Source: CAD feature listing. Evaluate the final solid. Frame: model axes, mm. A direction names the side the tool comes from. Coordinates: 2 decimals unless noted, no trailing zeros. Loops run counter-clockwise (first coordinate to the right, second up) from the corner with the lowest first, then second, coordinate; pieces in that order, holes last. Notation, with made-up numbers: (53.25, -39) - (96.25, -39) arc R27 cw to (96.25, -11) - close; hole circle Ø1 at (-2.5, 72). An arc over 180 degrees is marked (long way). Write item = value, one per line. Start each with the question number.
Autodesk Inventor part; units mm, degrees
ref_plane "YZ Plane" through (0, 0, 0) normal (1, 0, 0) x (0, 1, 0)
ref_plane "XZ Plane" through (0, 0, 0) normal (0, 1, 0) x (-1, 0, 0)
ref_plane "XY Plane" through (0, 0, 0) normal (0, 0, 1) x (1, 0, 0)
sketch "Sketch1" plane through (0, 0, 0) normal (0, 1, 0) x (-1, 0, 0)
  line L0 (0, 0) -> (70, 0)
  line L1 (70, 0) -> (70, -110)
  line L2 (70, -110) -> (0, -110)
  line L3 (0, -110) -> (0, 0)
  line L4 (2.5, -2.49) -> (67.5, -2.49)
  line L5 (67.5, -2.49) -> (67.5, -107.49)
  line L6 (67.5, -107.49) -> (2.5, -107.49)
  line L7 (2.5, -107.49) -> (2.5, -2.49)
  line L8 (67.5, -54.99) -> (2.5, -54.99) construction
  line L9 (67.5, -54.99) -> (63.6, -54.99) construction
  line L10 (63.6, -54.99) -> (63.6, -71.2) construction
  line L11 (63.6, -71.2) -> (67.5, -71.2) construction
  line L12 (67.5, -71.2) -> (67.5, -54.99) construction
  line L13 (63.6, -68.2) -> (63.6, -74.2) construction
  line L14 (62.35, -68.2) -> (62.35, -74.2)
  line L15 (64.85, -74.2) -> (64.85, -68.2)
  arc A0 (64.85, -68.2) -> (62.35, -68.2) centre (63.6, -68.2) ccw
  arc A1 (62.35, -74.2) -> (64.85, -74.2) centre (63.6, -74.2) ccw
  line L16 (63.6, -71.2) -> (63.6, -87.6) construction
  line L17 (2.5, -87.6) -> (6.05, -87.6) construction
  line L18 (6.05, -84.6) -> (6.05, -90.6) construction
  line L19 (4.8, -84.6) -> (4.8, -90.6)
  line L20 (7.3, -90.6) -> (7.3, -84.6)
  arc A2 (7.3, -84.6) -> (4.8, -84.6) centre (6.05, -84.6) ccw
  arc A3 (4.8, -90.6) -> (7.3, -90.6) centre (6.05, -90.6) ccw
  line L21 (67.5, -2.49) -> (63.6, -2.49) construction
  line L22 (63.6, -2.49) -> (63.6, -18.7) construction
  line L23 (63.6, -18.7) -> (67.5, -18.7) construction
  line L24 (67.5, -18.7) -> (67.5, -2.49) construction
  line L25 (63.6, -18.7) -> (63.6, -35.1) construction
  line L26 (2.5, -35.1) -> (6.05, -35.1) construction
  line L27 (63.6, -15.7) -> (63.6, -21.7) construction
  line L28 (62.35, -15.7) -> (62.35, -21.7)
  line L29 (64.85, -21.7) -> (64.85, -15.7)
  arc A4 (64.85, -15.7) -> (62.35, -15.7) centre (63.6, -15.7) ccw
  arc A5 (62.35, -21.7) -> (64.85, -21.7) centre (63.6, -21.7) ccw
  line L30 (6.05, -32.1) -> (6.05, -38.1) construction
  line L31 (4.8, -32.1) -> (4.8, -38.1)
  line L32 (7.3, -38.1) -> (7.3, -32.1)
  arc A6 (7.3, -32.1) -> (4.8, -32.1) centre (6.05, -32.1) ccw
  arc A7 (4.8, -38.1) -> (7.3, -38.1) centre (6.05, -38.1) ccw
  point P0 (35, -55)
  dimension "d0" = 70
  dimension "d1" = 110
  dimension "d2" = 65
  dimension "d3" = 105
  dimension "d4" = 52.5
  dimension "d5" = 52.5
  dimension "d6" = 3.9
  dimension "d7" = 16.21
  dimension "d8" = 3
  dimension "d9" = 2.5
  dimension "d10" = 16.4
  dimension "d11" = 3.55
  dimension "d12" = 3
  dimension "d13" = 2.5
  dimension "d14" = 19.89
  dimension "d15" = 16.4
  dimension "d16" = 3.9
  dimension "d17" = 16.21
  dimension "d18" = 16.4
  dimension "d19" = 3.55
  dimension "d20" = 3
  dimension "d21" = 2.5
  dimension "d22" = 3
  dimension "d23" = 2.5
extrude "Extrusion1" add sketch "Sketch1" along normal blind 25 contours L0 L1 L2 L3
extrude "Extrusion2" add sketch "Sketch1" along normal blind 5 contours L4 L5 L6 L7
sketch "Sketch2" plane through (0, 0, 0) normal (0, -1, 0) x (1, 0, 0)
  line L0 (-63.6, -21.7) -> (-63.6, -15.7) construction
  line L1 (-61.6, -21.7) -> (-61.6, -15.7)
  line L2 (-65.6, -15.7) -> (-65.6, -21.7)
  arc A0 (-65.6, -21.7) -> (-61.6, -21.7) centre (-63.6, -21.7) ccw
  arc A1 (-61.6, -15.7) -> (-65.6, -15.7) centre (-63.6, -15.7) ccw
  line L3 (-6.0099, -38.1033) -> (-6.0099, -32.1033) construction
  line L4 (-4.0099, -38.1033) -> (-4.0099, -32.1033)
  line L5 (-8.0099, -32.1033) -> (-8.0099, -38.1033)
  arc A2 (-8.0099, -38.1033) -> (-4.0099, -38.1033) centre (-6.0099, -38.1033) ccw
  arc A3 (-4.0099, -32.1033) -> (-8.0099, -32.1033) centre (-6.0099, -32.1033) ccw
  line L6 (-63.6, -74.2793) -> (-63.6, -68.2793) construction
  line L7 (-61.6, -74.2793) -> (-61.6, -68.2793)
  line L8 (-65.6, -68.2793) -> (-65.6, -74.2793)
  arc A4 (-65.6, -74.2793) -> (-61.6, -74.2793) centre (-63.6, -74.2793) ccw
  arc A5 (-61.6, -68.2793) -> (-65.6, -68.2793) centre (-63.6, -68.2793) ccw
  line L9 (-6.0099, -90.6) -> (-6.0099, -84.6) construction
  line L10 (-4.8, -90.6) -> (-4.8, -84.6)
  line L11 (-4.0099, -90.6) -> (-4.0099, -84.6)
  line L12 (-8.0099, -84.6) -> (-8.0099, -90.6)
  arc A6 (-8.0099, -90.6) -> (-4.0099, -90.6) centre (-6.0099, -90.6) ccw
  arc A7 (-4.0099, -84.6) -> (-8.0099, -84.6) centre (-6.0099, -84.6) ccw
  line L13 (-6.0099, -87.6) -> (-0.0099, -87.6) construction
  point P0 (0, 0)
  point P1 (-63.6, -18.7)
  point P2 (-6.0099, -35.1033)
  point P3 (-63.6, -71.2793)
  dimension "d28" = 3
  dimension "d29" = 4
  dimension "d30" = 3
  dimension "d31" = 4
  dimension "d32" = 3
  dimension "d33" = 4
  dimension "d34" = 3
  dimension "d35" = 90
  dimension "d36" = 4
extrude "Extrusion3" cut sketch "Sketch2" against normal blind 1
sketch "Sketch3" plane through (0, 25, 0) normal (0, 1, 0) x (1, 0, 0)
  line L0 (-67.5, 2.49) -> (-67.5, 107.49)
  circle A0 centre (-67.5, 2.49) radius 2.5
  line L1 (-70, 2) -> (-70, 108)
  circle A1 centre (-67.5, 107.477) radius 2.5
  line L2 (-67.5, 107.49) -> (-2.5, 107.49)
  circle A2 centre (-2.5, 107.49) radius 2.5
  point P0 (0, 0)
  dimension "d40" = 5
extrude "Extrusion4" add sketch "Sketch3" against normal blind 24 contours A2 | A0 | A1 L2 L0 | L0 L2 A1
sketch "Sketch5" plane through (0, 0, 0) normal (0, -1, 0) x (1, 0, 0)
  arc A0 (-2.5, -104.99) -> (-5, -107.49) centre (-2.5, -107.49) ccw
  arc A1 (-65, -107.49) -> (-67.5, -104.977) centre (-67.5, -107.477) ccw
  arc A2 (-67.5, -4.99) -> (-65, -2.49) centre (-67.5, -2.49) ccw
  point P0 (0, 0)
hole "Hole1" at (-2.5, 0, -107.49) at (-67.5, 0, -107.477) at (-67.5, 0, -2.49) direction (0, 1, 0) diameter 3 depth 40 tip angle 118 counterbore diameter 3.5 counterbore depth 2
fillet "Fillet2" radius 2 4 edges at (-70, 12.5, 0) (-70, 12.5, -110) (0, 12.5, -110) (0, 12.5, 0)
sketch "Sketch6" plane through (0, 0, 0) normal (0, -1, 0) x (1, 0, 0)
  line L0 (-19.0093, -31.0437) -> (-19.0093, -43.6077) construction
  line L1 (-19.0093, -43.6077) -> (-93.3266, -43.6077) construction
  line L2 (-93.3266, -43.6077) -> (-93.3266, -31.0437) construction
  line L3 (-93.3266, -31.0437) -> (-19.0093, -31.0437) construction
  line L4 (-32.1283, -26.5619) -> (-32.1283, -53.8239) construction
  line L5 (-32.1283, -53.8239) -> (-124.1375, -53.8239) construction
  line L6 (-124.1375, -53.8239) -> (-124.1375, -26.5619) construction
  line L7 (-124.1375, -26.5619) -> (-32.1283, -26.5619) construction
  line L8 (-45.7196, -50.7865) -> (-45.7196, -85.058) construction
  line L9 (-45.7196, -85.058) -> (-48.896, -85.058) construction
  line L10 (-48.896, -85.058) -> (-48.896, -50.7865) construction
  line L11 (-48.896, -50.7865) -> (-45.7196, -50.7865) construction
  point P0 (0, 0)
properties part number "SUPERIOR MODEL2"
Item 1: Cut plane C-C (x = -51.5). Return the cut outline in (y, z), then the cut area to 3 significant figures.
Item 2: Cut plane B-B (z = -88.5). Return the cut outline in (x, y), then the cut area to 3 significant figures.
Item 3: First-contact query: pin 1 (5 mm diameter, centred on x = -19.5, y = 9, fed in from +Z); pin 2 (12 mm diameter, centred on x = -52, z = -39.5, fed in from +Y); pin 3 (1.8 mm diameter, centred on x = -3, z = -108, fed in from -Y). Flat tips, straight axial feed; report the tip coordinate or a pass-through.
Item 4: Material intervals for L1, parallel to X at y = 0.75, z = -107.49; L2, parallel to Z at x = -11, y = 18; L3, parallel to X at y = 19.5, z = -74.5, sorted ascending. Write a range as [from, to].
Item 5: Draft query along X for faces 1 (the cylindrical face through (-69.4, 12.68, -109.43)), 2 (the cylindrical face through (-0.6, 12.68, -0.57)), 3 (the flat face through (-62.35, 3, -71)). Return one class per face: released by +X, released by -X, zero draft, split by the parting line, or undercut.
Item 6: Cut plane A-A (y = 9.75). Return the cut outline in (x, z), then the cut area to 3 significant figures.
Item 7: Cut plane D-D (z = -25). Return the cut outline in (x, y).
Item 8: Reachability of faces 4 (the cylindrical face through (-6, 0.5, -82.6)), 5 (the cylindrical face through (-65.75, 15.14, -105.69)), 6 (the flat face through (-4.8, 3, -35)) from +Z, -Z, +X, -X, +Y, -Y: full face, straight path, thin tool, end or side. Return the list, or none.
Responses:
q1.outline = (0, -110) - (25, -110) - (25, -107.49) - (5, -107.49) - (5, -2.49) - (25, -2.49) - (25, 0) - (0, 0) - close
q1.area = 650 mm2
q2.outline = (-70, 0) - (-8.01, 0) - (-8.01, 1) - (-7.3, 1) - (-7.3, 5) - (-67.5, 5) - (-67.5, 25) - (-70, 25) - close; (-4.8, 1) - (-4.01, 1) - (-4.01, 0) - (0, 0) - (0, 25) - (-2.5, 25) - (-2.5, 5) - (-4.8, 5) - close
q2.area = 436 mm2
q3.pin_1 = 0
q3.pin_2 = 5
q3.pin_3 = 2
q4.L1 = [-70, -69.25], [-65.75, -4.25], [-0.75, 0]
q4.L2 = [-110, -107.49], [-2.49, 0]
q4.L3 = [-70, -67.5], [-2.5, 0]
q5.face_1 = released by -X
q5.face_2 = released by +X
q5.face_3 = undercut
q6.outline = (-70, -108) arc R2 ccw to (-68, -110) - (-2, -110) arc R2 ccw to (0, -108) - (0, -2) arc R2 ccw to (-2, 0) - (-67.28, 0) arc R2.5 ccw to (-67.72, 0) - (-68, 0) arc R2 ccw to (-70, -2) - close; hole circle Ø3 at (-67.5, -107.48); hole circle Ø3 at (-67.5, -2.49); hole (-67.5, -104.98) arc R2.5 cw to (-65, -107.49) - (-5, -107.49) arc R2.5 cw to (-2.5, -104.99) - (-2.5, -2.49) - (-65, -2.49) arc R2.5 cw to (-67.5, -4.99) - close; hole circle Ø3 at (-2.5, -107.49)
q6.area = 865 mm2
q7.outline = (-70, 0) - (0, 0) - (0, 25) - (-2.5, 25) - (-2.5, 5) - (-67.5, 5) - (-67.5, 25) - (-70, 25) - close
q8.face_4 = -Y
q8.face_5 = +Y
q8.face_6 = +Y, -Y
